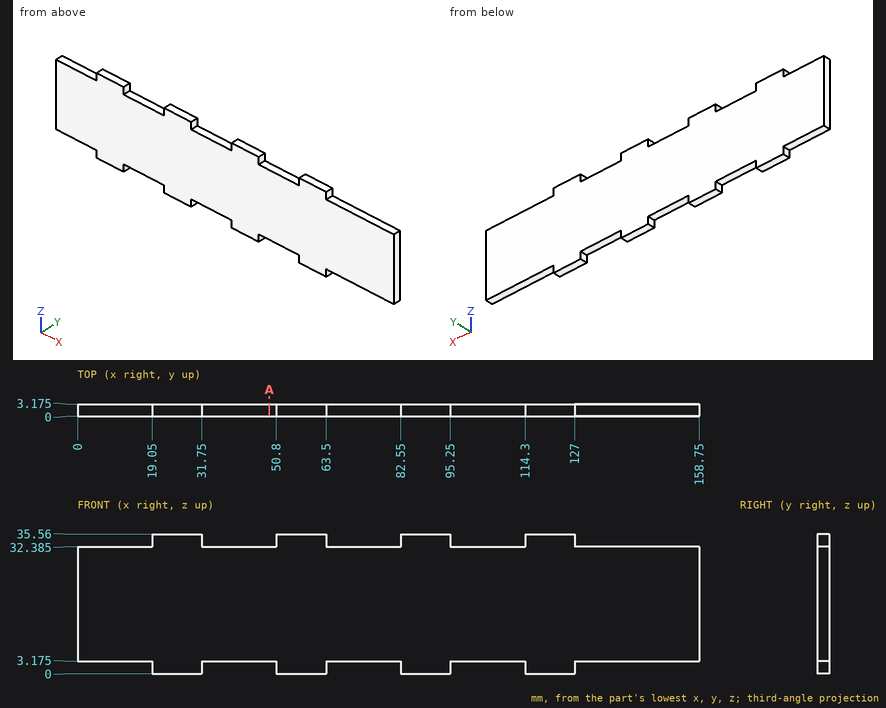
Geometry: see drawing. Coordinates: mm, zero at the bounding-box minimum. Give positions to 0.01 mm unless a question says otherwise; leave off trailing zeros. Order: outer loops, then holes, each group sorted by start corner. A loop starts at its lowest first (then second) coordinate and runs counter-clockwise, first axis right, second up.
Q1. Section A-A on x = 49. Output: boundary loops of the cut face in (y, z) (3 decimals).
Checked values:
outline: (0, 3.175) - (3.175, 3.175) - (3.175, 32.385) - (0, 32.385) - close
Q2. Ray query, probe 1 along Z at (x, y) = (38, 1.65) (3 decimals). Return the intervals inside material, ascending.
Checked values:
probe 1: z = 3.175 to 32.385
Q3. Contact query for flat-ended pins moving along their axis: pin 1 Ø1 at (x, y) = (109.5, 1) entering from +Z (3 decimals); pin 2 Ø1 at (y, z) = (2, 33.5) entering from +X; pin 3 Ø1 at (y, z) = (1, 1) entering from -X. Output: stop coordinate, or through.
Checked values:
pin 1: stops at z = 32.385
pin 2: stops at x = 127
pin 3: stops at x = 19.05
